Read the model definition and answer for the solid it produces. Units are mm, in the model's axes. Face numbers are marked on the shaded views. Round coordinates to 2 decimals unless told otherwise and drop trailing zeros. Use CSV: the item, a comma, the result in double quotes. Start each with the question number.
1. Given pin 1 Ø4 at (x, z) = (2, -14.5) entering from +Y, flat-ended and moving along its own axis, determine where the tip first touches the part or whether it passes through.
2. Consider line 1 along X through (y, z) = (2, 0); line 2 along Z through (x, y) = (30.5, -2.1); line 3 along X through (y, z) = (1.1, -36). Determine where each line is inside the solid, lowest interval first.
3. Determine the mould class of the marked faces 1 and 2 for opening direction Z: +Z half, -Z half, draft (parallel to the pull), parting line (faces both ways), or undercut.
4. Find section A-A (x = -29). State how many separate pieces and enclosed holes the cut face has, and give its area (3 significant figures).
from build123d import *

# Parameters (mm, degrees)
SKETCH_2_R          = 52.5
SKETCH_2_R_2        = 2.65
EXTRUDE_1_DEPTH     = 2.75
SKETCH_3_R          = 54
SKETCH_3_R_2        = 52.5
EXTRUDE_2_DEPTH     = 1
SKETCH_4_R          = 50
SKETCH_4_R_2        = 2.65
CUT_EXTRUDE_1_DEPTH = 1
FILLET_1_R          = 1.5


with BuildPart() as part:
    # 草图2 → 凸台-拉伸1 (new, symmetric)
    with BuildSketch(Plane(origin=(0, 0, 0), x_dir=(1, 0, 0), z_dir=(0, 1, 0))):
        with Locations(Location((0, 0, 0), (0, 0, 270))):
            Circle(SKETCH_2_R)
        with Locations(Location((0, 0, 0), (0, 0, 270))):
            Circle(SKETCH_2_R_2, mode=Mode.SUBTRACT)
        with BuildLine():
            Line((-5.104760308, -3.608479293), (-30.908533356, -33.241423952))
            ThreePointArc((-30.908533356, -33.241423952), (-32.355479798, -33.927082172), (-33.841752753, -33.331453173))
            ThreePointArc((-33.841752753, -33.331453173), (-45.175184524, -14.678307233), (-46.970289709, 7.074028884))
            ThreePointArc((-46.970289709, 7.074028884), (-46.117971572, 8.42951219), (-44.544347521, 8.725296818))
            Line((-44.544347521, 8.725296818), (-6.250848753, -0.081181754))
            ThreePointArc((-6.250848753, -0.081181754), (-5.333939805, -0.568676849), (-4.785067523, -1.450216811))
            ThreePointArc((-4.785067523, -1.450216811), (-4.755282581, -1.545084972), (-4.723617, -1.639342075))
            ThreePointArc((-4.723617, -1.639342075), (-4.649507815, -2.675141919), (-5.104760308, -3.608479293))
        make_face(mode=Mode.SUBTRACT)
        with BuildLine():
            Line((-5.009325433, 3.73983413), (-41.165734939, 19.123597139))
            ThreePointArc((-41.165734939, 19.123597139), (-42.264965697, 20.287844939), (-42.157772458, 21.885434001))
            ThreePointArc((-42.157772458, 21.885434001), (-27.919799484, 38.428307233), (-7.786816484, 46.857395244))
            ThreePointArc((-7.786816484, 46.857395244), (-6.234294464, 46.465659903), (-5.466709992, 45.060456971))
            Line((-5.466709992, 45.060456971), (-2.00882693, 5.919823897))
            ThreePointArc((-2.00882693, 5.919823897), (-2.18912187, 4.897147398), (-2.857905332, 4.102728009))
            ThreePointArc((-2.857905332, 4.102728009), (-2.938926261, 4.045084972), (-3.018784891, 3.985842167))
            ThreePointArc((-3.018784891, 3.985842167), (-3.980988084, 3.595280389), (-5.009325433, 3.73983413))
        make_face(mode=Mode.SUBTRACT)
        with BuildLine():
            Line((1.854410058, -5.96999698), (22.063210783, -39.667926976))
            ThreePointArc((22.063210783, -39.667926976), (22.26817946, -41.255934861), (21.242419017, -42.485404956))
            ThreePointArc((21.242419017, -42.485404956), (0, -47.5), (-21.242419017, -42.485404956))
            ThreePointArc((-21.242419017, -42.485404956), (-22.26817946, -41.255934861), (-22.063210783, -39.667926976))
            Line((-22.063210783, -39.667926976), (-1.854410058, -5.96999698))
            ThreePointArc((-1.854410058, -5.96999698), (-1.107434224, -5.24860902), (-0.099429036, -4.999011289))
            ThreePointArc((-0.099429036, -4.999011289), (0, -5), (0.099429036, -4.999011289))
            ThreePointArc((0.099429036, -4.999011289), (1.107434224, -5.24860902), (1.854410058, -5.96999698))
        make_face(mode=Mode.SUBTRACT)
        with BuildLine():
            Line((6.250848753, -0.081181754), (44.544347521, 8.725296818))
            ThreePointArc((44.544347521, 8.725296818), (46.117971572, 8.42951219), (46.970289709, 7.074028884))
            ThreePointArc((46.970289709, 7.074028884), (45.175184524, -14.678307233), (33.841752753, -33.331453173))
            ThreePointArc((33.841752753, -33.331453173), (32.355479798, -33.927082172), (30.908533356, -33.241423952))
            Line((30.908533356, -33.241423952), (5.104760308, -3.608479293))
            ThreePointArc((5.104760308, -3.608479293), (4.649507815, -2.675141919), (4.723617, -1.639342075))
            ThreePointArc((4.723617, -1.639342075), (4.755282581, -1.545084972), (4.785067523, -1.450216811))
            ThreePointArc((4.785067523, -1.450216811), (5.333939805, -0.568676849), (6.250848753, -0.081181754))
        make_face(mode=Mode.SUBTRACT)
        with BuildLine():
            Line((2.00882693, 5.919823897), (5.466709992, 45.060456971))
            ThreePointArc((5.466709992, 45.060456971), (6.234294464, 46.465659903), (7.786816484, 46.857395244))
            ThreePointArc((7.786816484, 46.857395244), (27.919799484, 38.428307233), (42.157772458, 21.885434001))
            ThreePointArc((42.157772458, 21.885434001), (42.264965697, 20.287844939), (41.165734939, 19.123597139))
            Line((41.165734939, 19.123597139), (5.009325433, 3.73983413))
            ThreePointArc((5.009325433, 3.73983413), (3.980988084, 3.595280389), (3.018784891, 3.985842167))
            ThreePointArc((3.018784891, 3.985842167), (2.938926261, 4.045084972), (2.857905332, 4.102728009))
            ThreePointArc((2.857905332, 4.102728009), (2.18912187, 4.897147398), (2.00882693, 5.919823897))
        make_face(mode=Mode.SUBTRACT)
    extrude(amount=EXTRUDE_1_DEPTH, both=True)

    # 草图3 → 凸台-拉伸2 (add)
    with BuildSketch(Plane(origin=(0, 2.75, 0), x_dir=(1, 0, 0), z_dir=(0, 1, 0))):
        with Locations(Location((0, 0, 0), (0, 0, 270))):
            Circle(SKETCH_3_R)
        with Locations(Location((0, 0, 0), (0, 0, 270))):
            Circle(SKETCH_3_R_2, mode=Mode.SUBTRACT)
    extrude_2 = extrude(amount=-EXTRUDE_2_DEPTH)

    # 草图4 → 切除-拉伸1 (cut)
    with BuildSketch(Plane(origin=(0, 2.75, 0), x_dir=(1, 0, 0), z_dir=(0, 1, 0))):
        with Locations(Location((0, 0, 0), (0, 0, 270))):
            Circle(SKETCH_4_R)
        with Locations(Location((0, 0, 0), (0, 0, 270))):
            Circle(SKETCH_4_R_2, mode=Mode.SUBTRACT)
        with BuildLine():
            Line((41.165734939, 19.123597139), (5.009325433, 3.73983413))
            ThreePointArc((5.009325433, 3.73983413), (3.980988084, 3.595280389), (3.018784891, 3.985842167))
            ThreePointArc((3.018784891, 3.985842167), (2.938926261, 4.045084972), (2.857905332, 4.102728009))
            ThreePointArc((2.857905332, 4.102728009), (2.18912187, 4.897147398), (2.00882693, 5.919823897))
            Line((2.00882693, 5.919823897), (5.466709992, 45.060456971))
            ThreePointArc((5.466709992, 45.060456971), (6.234294464, 46.465659903), (7.786816484, 46.857395244))
            ThreePointArc((7.786816484, 46.857395244), (27.919799484, 38.428307233), (42.157772458, 21.885434001))
            ThreePointArc((42.157772458, 21.885434001), (42.264965697, 20.287844939), (41.165734939, 19.123597139))
        make_face(mode=Mode.SUBTRACT)
        with BuildLine():
            Line((30.908533356, -33.241423952), (5.104760308, -3.608479293))
            ThreePointArc((5.104760308, -3.608479293), (4.649507815, -2.675141919), (4.723617, -1.639342075))
            ThreePointArc((4.723617, -1.639342075), (4.755282581, -1.545084972), (4.785067523, -1.450216811))
            ThreePointArc((4.785067523, -1.450216811), (5.333939805, -0.568676849), (6.250848753, -0.081181754))
            Line((6.250848753, -0.081181754), (44.544347521, 8.725296818))
            ThreePointArc((44.544347521, 8.725296818), (46.117971572, 8.42951219), (46.970289709, 7.074028884))
            ThreePointArc((46.970289709, 7.074028884), (45.175184524, -14.678307233), (33.841752753, -33.331453173))
            ThreePointArc((33.841752753, -33.331453173), (32.355479798, -33.927082172), (30.908533356, -33.241423952))
        make_face(mode=Mode.SUBTRACT)
        with BuildLine():
            Line((-22.063210783, -39.667926976), (-1.854410058, -5.96999698))
            ThreePointArc((-1.854410058, -5.96999698), (-1.107434224, -5.24860902), (-0.099429036, -4.999011289))
            ThreePointArc((-0.099429036, -4.999011289), (0, -5), (0.099429036, -4.999011289))
            ThreePointArc((0.099429036, -4.999011289), (1.107434224, -5.24860902), (1.854410058, -5.96999698))
            Line((1.854410058, -5.96999698), (22.063210783, -39.667926976))
            ThreePointArc((22.063210783, -39.667926976), (22.26817946, -41.255934861), (21.242419017, -42.485404956))
            ThreePointArc((21.242419017, -42.485404956), (0, -47.5), (-21.242419017, -42.485404956))
            ThreePointArc((-21.242419017, -42.485404956), (-22.26817946, -41.255934861), (-22.063210783, -39.667926976))
        make_face(mode=Mode.SUBTRACT)
        with BuildLine():
            Line((-44.544347521, 8.725296818), (-6.250848753, -0.081181754))
            ThreePointArc((-6.250848753, -0.081181754), (-5.333939805, -0.568676849), (-4.785067523, -1.450216811))
            ThreePointArc((-4.785067523, -1.450216811), (-4.755282581, -1.545084972), (-4.723617, -1.639342075))
            ThreePointArc((-4.723617, -1.639342075), (-4.649507815, -2.675141919), (-5.104760308, -3.608479293))
            Line((-5.104760308, -3.608479293), (-30.908533356, -33.241423952))
            ThreePointArc((-30.908533356, -33.241423952), (-32.355479798, -33.927082172), (-33.841752753, -33.331453173))
            ThreePointArc((-33.841752753, -33.331453173), (-45.175184524, -14.678307233), (-46.970289709, 7.074028884))
            ThreePointArc((-46.970289709, 7.074028884), (-46.117971572, 8.42951219), (-44.544347521, 8.725296818))
        make_face(mode=Mode.SUBTRACT)
        with BuildLine():
            ThreePointArc((-7.786816484, 46.857395244), (-6.234294464, 46.465659903), (-5.466709992, 45.060456971))
            Line((-5.466709992, 45.060456971), (-2.00882693, 5.919823897))
            ThreePointArc((-2.00882693, 5.919823897), (-2.18912187, 4.897147398), (-2.857905332, 4.102728009))
            ThreePointArc((-2.857905332, 4.102728009), (-2.938926261, 4.045084972), (-3.018784891, 3.985842167))
            ThreePointArc((-3.018784891, 3.985842167), (-3.980988084, 3.595280389), (-5.009325433, 3.73983413))
            Line((-5.009325433, 3.73983413), (-41.165734939, 19.123597139))
            ThreePointArc((-41.165734939, 19.123597139), (-42.264965697, 20.287844939), (-42.157772458, 21.885434001))
            ThreePointArc((-42.157772458, 21.885434001), (-27.919799484, 38.428307233), (-7.786816484, 46.857395244))
        make_face(mode=Mode.SUBTRACT)
    extrude(amount=-CUT_EXTRUDE_1_DEPTH, mode=Mode.SUBTRACT)

    # 镜向1: 凸台-拉伸2 across plane
    add(extrude_2.mirror(Plane.ZX))

    # 圆角1
    fillet_1_edges = [part.edges().sort_by_distance(p)[0] for p in [
        (0, 1.75, -52.5),
        (0, -1.75, -52.5),
    ]]
    fillet(fillet_1_edges, radius=FILLET_1_R - 0.0001)  # a hair under: the kernel refuses the full size


solid = part.part
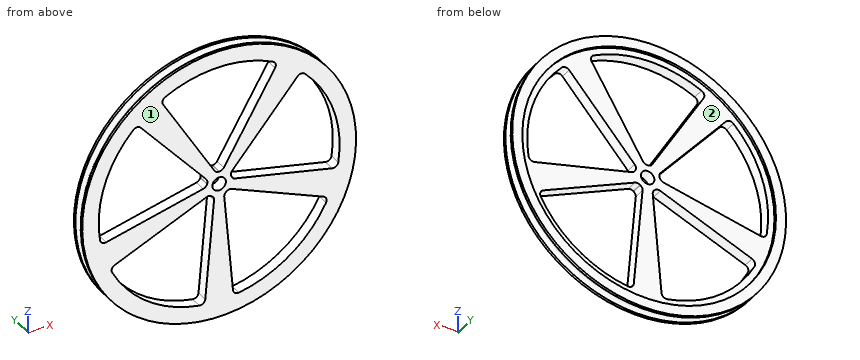
Filled sheet:
1,pin 1,"stops at y = 1.75"
2,line 1,"x = -54 to -50, 50 to 54"
2,line 2,"z = -44.56 to -36.41, -14.59 to -5.5, 32.77 to 44.56"
2,line 3,"x = -38.58 to -30.99, -4.67 to 4.67, 30.99 to 38.58"
3,face 1,"draft"
3,face 2,"undercut"
4,separate pieces,"3"
4,enclosed holes,"0"
4,area,"140 mm²"
